Check sheet for the modelled part. Datum: model origin and axes. Units: mm. A direction names the side the tool comes from. Give positions to 0.01 mm unless a question says otherwise; leave off trailing zeros. Write each question's results on one line, items separated by ' | '. Start each with the question number.
1. Tool access check on faces 1 (the face through (0, 257, -4)), 2 (the face through (10, 257, -6)), 3 (the face through (0, 257, 4)), 4 (the face through (6, 257, -10)), 5 (the face through (4, 257, 0)). Record the directions out of +Z, -Z, +X, -X, +Y, -Y that give a thin tool (end or side, any length) a straight path to the whole face; none if there is none.
2. Material ranges on L1, parallel to X at y = 224.5, z = 0; L2, parallel to X at y = 256.5, z = 6.25; L3, parallel to X at y = 166, z = 6, recorded low to high. Write a range as from..to.
3. Mould release check, pull along Z, two halves, no side actions. Record for faces 6 (the face through (-4, 257, 0)), 7 (the face through (-10, 257, -6)), 8 (the face through (-6, 257, -10)): +Z half, -Z half, draft (parallel to the pull), parting line (faces both ways), or undercut.
4. Gauge pin test, flat ends, axial feed: pin 1 Ø1.7 at (x, y) = (1.5, 267.5) entering from -Z; pin 2 Ø1.6 at (y, z) = (333, 0.5) entering from +X; pin 3 Ø3 at (x, y) = (-1, 243.5) entering from +Z. Record the tip position at first contact, or that the pin passes through.
from build123d import *

# Parameters (mm, degrees)
SKETCH1_R           = 2.1
BOSS_EXTRUDE1_DEPTH = 330


with BuildPart() as part:
    # Sketch1 → Boss-Extrude1 (new body)
    with BuildSketch(Plane(origin=(0, 420, 0), x_dir=(1, 0, 0), z_dir=(0, 1, 0))):
        with BuildLine():
            Line((4, 2.746364236), (8, 6.746364236))
            Line((8, 6.746364236), (8, 3))
            Line((8, 3), (10, 3))
            Line((10, 3), (10, 9.5))
            ThreePointArc((10, 9.5), (9.853553391, 9.853553391), (9.5, 10))
            Line((9.5, 10), (3, 10))
            Line((3, 10), (3, 8))
            Line((3, 8), (6.863334179, 8))
            Line((6.863334179, 8), (2.863334179, 4))
            Line((2.863334179, 4), (-2.75, 4))
            Line((-2.75, 4), (-6.75, 8))
            Line((-6.75, 8), (-3, 8))
            Line((-3, 8), (-3, 10))
            Line((-3, 10), (-9.5, 10))
            ThreePointArc((-9.5, 10), (-9.853553391, 9.853553391), (-10, 9.5))
            Line((-10, 9.5), (-10, 3))
            Line((-10, 3), (-8, 3))
            Line((-8, 3), (-8, 6.75))
            Line((-8, 6.75), (-4, 2.75))
            Line((-4, 2.75), (-4, -2.75))
            Line((-4, -2.75), (-8, -6.75))
            Line((-8, -6.75), (-8, -3))
            Line((-8, -3), (-10, -3))
            Line((-10, -3), (-10, -9.5))
            ThreePointArc((-10, -9.5), (-9.853553391, -9.853553391), (-9.5, -10))
            Line((-9.5, -10), (-3, -10))
            Line((-3, -10), (-3, -8))
            Line((-3, -8), (-6.75, -8))
            Line((-6.75, -8), (-2.75, -4))
            Line((-2.75, -4), (2.868469119, -4))
            Line((2.868469119, -4), (6.868469119, -8))
            Line((6.868469119, -8), (3, -8))
            Line((3, -8), (3, -10))
            Line((3, -10), (9.5, -10))
            ThreePointArc((9.5, -10), (9.853553391, -9.853553391), (10, -9.5))
            Line((10, -9.5), (10, -3))
            Line((10, -3), (8, -3))
            Line((8, -3), (8, -6.665189266))
            Line((8, -6.665189266), (4, -2.665189266))
            Line((4, -2.665189266), (4, 2.746364236))
        make_face()
        Circle(SKETCH1_R, mode=Mode.SUBTRACT)
    extrude(amount=-BOSS_EXTRUDE1_DEPTH)


solid = part.part
Geometry says:
1) face 1: -Z, +Y, -Y | face 2: +Z, -Z, +X, +Y, -Y | face 3: +Z, +Y, -Y | face 4: -Z, +X, -X, +Y, -Y | face 5: +X, +Y, -Y
2) L1: -4..-2.1, 2.1..4 | L2: -10..-8, -7.5..-5, 5.12..7.58, 8..10 | L3: -10..-8, -7.25..-4.75, 4.87..7.33, 8..10
3) face 6: undercut | face 7: draft | face 8: -Z half
4) pin 1: z = -4 | pin 2: x = 4 | pin 3: z = 4
